```python
from build123d import *

# Parameters (mm, degrees)
SKETCH002_R           = 3
POCKET_DEPTH          = 283.449725
POLARPATTERN_COUNT    = 6
POCKET001_DEPTH       = 5
POCKET002_DEPTH       = 5
POCKET003_DEPTH       = 5
POCKET004_DEPTH       = 13
POCKET005_DEPTH       = 13
POLARPATTERN001_COUNT = 6


with BuildPart() as part:
    # Sketch → Revolution (revolve)
    with BuildSketch(Plane.XY):
        Polygon((68.911188, 34), (68.911188, 31.5), (76.544998, 27.940296), (76.544998, 14.5), (81.044998, 14.5), (81.044998, 12.5), (104.911188, 12.5), (104.911188, 17), (103.911188, 17), (103.911188, 23.5), (81.911188, 23.5), (81.911188, 30.5), (76.911188, 30.5), (76.911188, 47), (72.411188, 47), (72.411188, 34), align=None)
    revolve(axis=Axis((0, 0, 0), (1, 0, 0)))

    # Sketch002 (on Face13 of Revolution) → Pocket (cut, through all)
    with BuildSketch(Plane.YZ.offset(76.911188)):
        with Locations((0, 40.5)):
            Circle(SKETCH002_R)
    pocket = extrude(amount=-POCKET_DEPTH, mode=Mode.SUBTRACT)

    # PolarPattern: Pocket ×6 about axis
    polarpattern_axis = Axis((76.911188, 0, 0), (1, 0, 0))
    for i in range(1, POLARPATTERN_COUNT):
        add(pocket.rotate(polarpattern_axis, i * 360 / POLARPATTERN_COUNT), mode=Mode.SUBTRACT)

    # Sketch006 (on Face19 of PolarPattern) → Pocket001 (cut)
    with BuildSketch(Plane.YZ.offset(104.911188)):
        with BuildLine():
            Line((-4.87718, 16.285365), (-6.849063, 22.479776))
            ThreePointArc((6.271238, 22.647772), (-0.30141, 23.53977), (-6.849063, 22.479776))
            Line((6.271238, 22.647772), (4.359747, 16.63002))
            ThreePointArc((4.359747, 16.63002), (-0.288728, 17.262036), (-4.87718, 16.285365))
        make_face()
    extrude(amount=-POCKET001_DEPTH, mode=Mode.SUBTRACT)

    # Sketch006 (on Face19 of PolarPattern) → Pocket002 (cut)
    with BuildSketch(Plane.YZ.offset(104.911188)):
        with BuildLine():
            Line((-4.87718, 16.285365), (-6.849063, 22.479776))
            ThreePointArc((6.271238, 22.647772), (-0.30141, 23.53977), (-6.849063, 22.479776))
            Line((6.271238, 22.647772), (4.359747, 16.63002))
            ThreePointArc((4.359747, 16.63002), (-0.288728, 17.262036), (-4.87718, 16.285365))
        make_face()
    extrude(amount=-POCKET002_DEPTH, mode=Mode.SUBTRACT)

    # Sketch006 (on Face19 of PolarPattern) → Pocket003 (cut)
    with BuildSketch(Plane.YZ.offset(104.911188)):
        with BuildLine():
            Line((-4.87718, 16.285365), (-6.849063, 22.479776))
            ThreePointArc((6.271238, 22.647772), (-0.30141, 23.53977), (-6.849063, 22.479776))
            Line((6.271238, 22.647772), (4.359747, 16.63002))
            ThreePointArc((4.359747, 16.63002), (-0.288728, 17.262036), (-4.87718, 16.285365))
        make_face()
    extrude(amount=-POCKET003_DEPTH, mode=Mode.SUBTRACT)

    # Sketch006 (on Face19 of PolarPattern) → Pocket004 (cut)
    with BuildSketch(Plane.YZ.offset(104.911188)):
        with BuildLine():
            Line((-4.87718, 16.285365), (-6.849063, 22.479776))
            ThreePointArc((6.271238, 22.647772), (-0.30141, 23.53977), (-6.849063, 22.479776))
            Line((6.271238, 22.647772), (4.359747, 16.63002))
            ThreePointArc((4.359747, 16.63002), (-0.288728, 17.262036), (-4.87718, 16.285365))
        make_face()
    extrude(amount=-POCKET004_DEPTH, mode=Mode.SUBTRACT)

    # Sketch006 (on Face19 of PolarPattern) → Pocket005 (cut)
    with BuildSketch(Plane.YZ.offset(104.911188)):
        with BuildLine():
            Line((-4.87718, 16.285365), (-6.849063, 22.479776))
            ThreePointArc((6.271238, 22.647772), (-0.30141, 23.53977), (-6.849063, 22.479776))
            Line((6.271238, 22.647772), (4.359747, 16.63002))
            ThreePointArc((4.359747, 16.63002), (-0.288728, 17.262036), (-4.87718, 16.285365))
        make_face()
    pocket005 = extrude(amount=-POCKET005_DEPTH, mode=Mode.SUBTRACT)

    # PolarPattern001: Pocket005 ×6 about axis
    polarpattern001_axis = Axis((104.911188, 0, 0), (1, 0, 0))
    for i in range(1, POLARPATTERN001_COUNT):
        add(pocket005.rotate(polarpattern001_axis, i * 360 / POLARPATTERN001_COUNT), mode=Mode.SUBTRACT)


solid = part.part
```
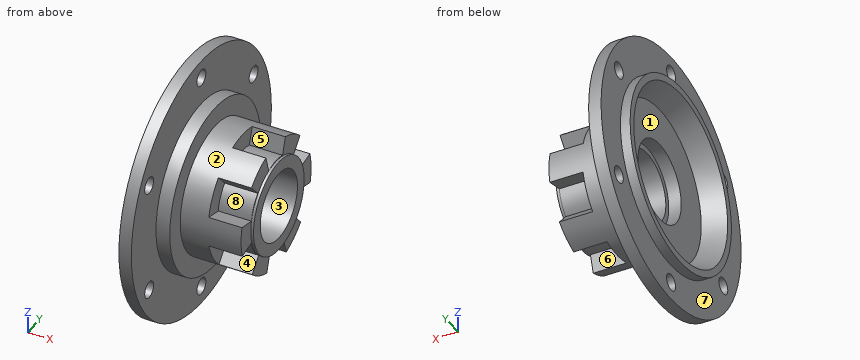
Check sheet for the modelled part. Datum: model origin and axes. Units: mm. Face numbers are marked on the shaded views. A direction names the side the tool comes from. Coordinates: 2 decimals unless noted, no trailing zeros. Write each loop counter-clockwise with the first axis right and the second up, starting at its lowest first coordinate (ties: lowest second). Pieces come first, ordered by that corner, then holes. Notation, with made-up numbers: (67, 15.5) - (104, 15.5) arc R19 ccw to (104, 39.5) - close; hole circle Ø7 at (36.5, 2). An arc over 180 degrees is marked (long way). One line per question, with ' | ' between items.
Item 1: Gauge pin test, flat ends, axial feed: P1, Ø1, axis at x = 95, z = 13.5, coming from the +Y side; P2, Ø6, axis at x = 89.5, z = -8.5, coming from the -Y side; P3, Ø12, axis at y = 26, z = -9, coming from the +X side; P4, Ø3, axis at y = 1, z = 17, coming from the +X side. Record the tip position at first contact, or that the pin passes through.
Determined:
P1: stops at y = 13.15 | P2: stops at y = -22.85 | P3: stops at x = 103.91 | P4: stops at x = 104.91
Item 2: Thickness scan on line 1 (Y direction, x = 75, z = 20); line 2 (Y direction, x = 75.5, z = 23); line 3 (Z direction, x = 74.1, y = 0). Record the ranges inside material, lowest first. Write a range as [from, to].
Determined:
line 1: y = [-42.53, -38.06], [-32.08, -20.53], [20.53, 32.08], [38.06, 42.53] | line 2: y = [-40.99, -36.27], [-33.88, -16.71], [16.71, 33.88], [36.27, 40.99] | line 3: z = [-47, -43.5], [-37.5, -29.08], [29.08, 37.5], [43.5, 47]
Item 3: Access from +Z, -Z, +X, -X, +Y, -Y to the whole of each face (thin tool, end or side, straight path). Record for the marked faces 1, 2, 3 and 4.
Determined:
face 1: -X | face 2: +X | face 3: +X, -X | face 4: +X, -Y
Item 4: Sectioned sample at C-C on y = 0. Give the number of separate pieces and of enclosed holes in the cut face, plus the area to 3 significant figures.
Determined:
separate pieces: 4 | enclosed holes: 0 | area: 650 mm2
Item 5: Mould release check, pull along Z, two halves, no side actions. Record for the marked faces 5, 6, 7 and 8: pulls with the +Z half, pulls with the -Z half, needs draft (parallel to the pull), parting line crosses it, or undercut.
Determined:
face 5: pulls with the +Z half | face 6: pulls with the -Z half | face 7: needs draft | face 8: undercut
Item 6: Sectioned sample at D-D on x = 89. Record the boundary of the cut face in (y, z).
Determined:
outline: circle Ø47 at (0, 0); hole circle Ø25 at (0, 0)
Item 7: Sectioned sample at A-A on x = 97. Record the boundary of the cut face in (y, z).
Determined:
outline: (-22.89, 5.31) arc R23.5 ccw to (-22.75, -5.89) - (-16.58, -4.54) arc R13.67 ccw to (-11.66, -12.37) - (-16.04, -17.17) arc R23.5 ccw to (-6.27, -22.65) - (-4.36, -16.63) arc R13.67 ccw to (4.88, -16.29) - (6.85, -22.48) arc R23.5 ccw to (16.48, -16.75) - (12.22, -12.09) arc R13.67 ccw to (16.54, -3.92) - (22.89, -5.31) arc R23.5 ccw to (22.75, 5.89) - (16.58, 4.54) arc R13.67 ccw to (11.66, 12.37) - (16.04, 17.17) arc R23.5 ccw to (6.27, 22.65) - (4.36, 16.63) arc R13.67 ccw to (-4.88, 16.29) - (-6.85, 22.48) arc R23.5 ccw to (-16.48, 16.75) - (-12.22, 12.09) arc R13.67 ccw to (-16.54, 3.92) - close; hole circle Ø25 at (0, 0)
